Here's the drawing with two shaded views (mm, measured from the low corner). I have some questions. A direction names the side the tool comes from. Give positions to 0.01 mm unless a question says otherwise; leave off trailing zeros. Loops run counter-clockwise (first coordinate to the right, second up) from the corner with the lowest first, then second, coordinate; pieces in that order, holes last. Notation, with made-up numbers: (52.5, 60) - (65.5, 60) arc R14 ccw to (65.5, 74) - close; hole circle Ø7 at (27, -5). An arc over 180 degrees is marked (long way). Write each question's results on one line, items separated by ' | '. Start each with the question number.
1) If we mould it in two halves opening along Y, with no side actions, what happens to the marked faces 3, 4 and 5? For each: +Y half, -Y half, draft (parallel to the pull), parting line (faces both ways), or undercut.
2) If I drill on probe 1 along Y at (x, z) = (21.5, 28); probe 2 along Z at (x, y) = (9, 15.75), over which ranges is the centre line in solid material (lowest first)? Write a range as [from, to].
3) I want a section at A-A, the plane z = 27.5. Write out the boundary of the cut face in (x, y), and give its area (3 significant figures).
4) I'm going to push a flat-ended pin straight in: pin 1 (4 mm diameter, centred on x = 8.5, y = 11.5, fed in from +Z). Where does the tip first touch, or does it pass through?
5) I want a section at C-C, the plane y = 11.25. Write out the boundary of the cut face in (x, z), and give its area (3 significant figures).
6) I want a section at B-B, the plane x = 23. Write out the boundary of the cut face in (y, z), and give its area (3 significant figures).
7) On a 3-axis mill with a long thin cutter (end or side, diameter ignored), from which of +Z, -Z, +X, -X, +Y, -Y can I reach the whole of each face in a straight line? I mean the marked faces 1 and 2. Say none if no direction works.
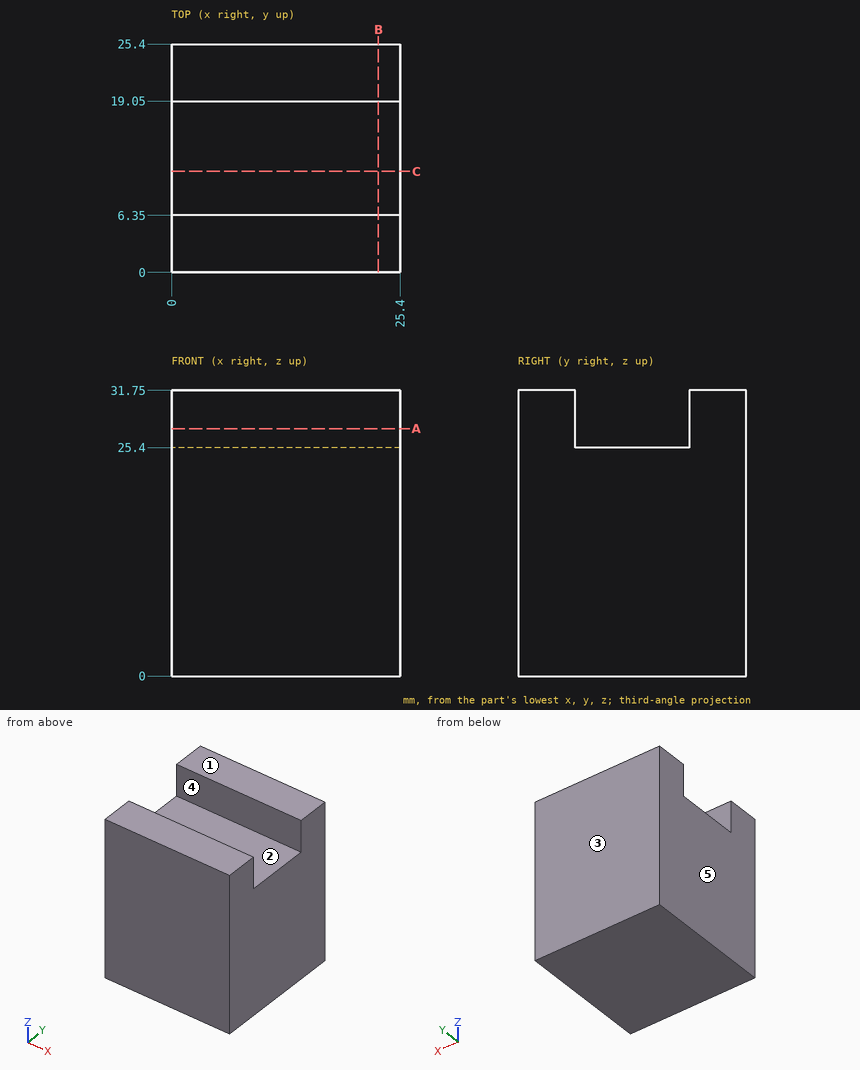
Answers:
1) face 3: +Y half | face 4: undercut | face 5: draft
2) probe 1: y = [0, 6.35], [19.05, 25.4] | probe 2: z = [0, 25.4]
3) outline: (0, 0) - (25.4, 0) - (25.4, 6.35) - (0, 6.35) - close; (0, 19.05) - (25.4, 19.05) - (25.4, 25.4) - (0, 25.4) - close | area: 323 mm2
4) pin 1: stops at z = 25.4
5) outline: (0, 0) - (25.4, 0) - (25.4, 25.4) - (0, 25.4) - close | area: 645 mm2
6) outline: (0, 0) - (25.4, 0) - (25.4, 31.75) - (19.05, 31.75) - (19.05, 25.4) - (6.35, 25.4) - (6.35, 31.75) - (0, 31.75) - close | area: 726 mm2
7) face 1: +Z, +X, -X, +Y, -Y | face 2: +Z, +X, -X
